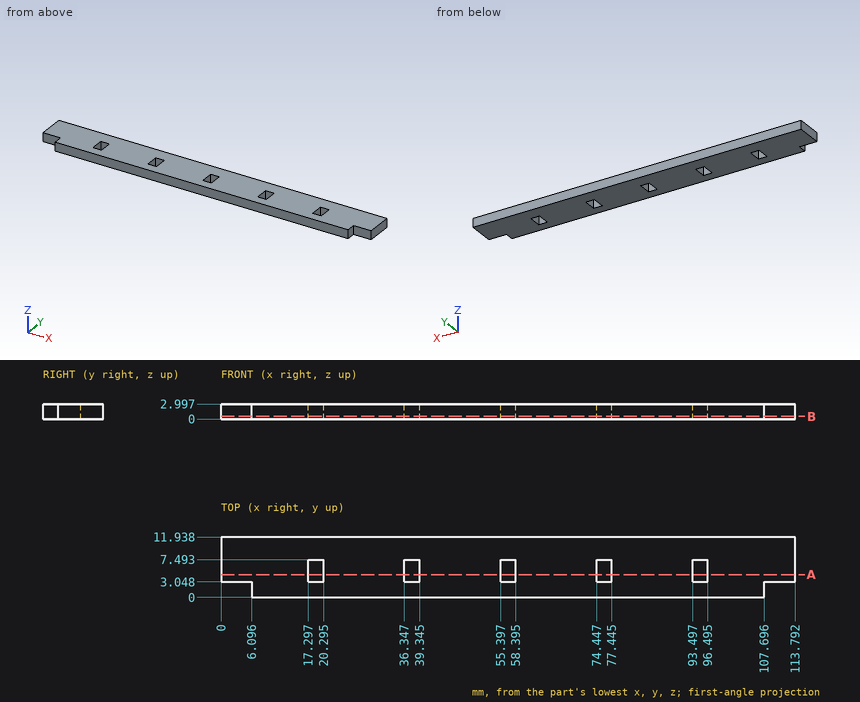
Here's the drawing with two shaded views (mm, measured from the low corner). I have some questions. Give positions to 0.01 mm unless a question says otherwise; leave off trailing zeros. Loops run counter-clockwise (first coordinate to the right, second up) from the corner with the lowest first, then second, coordinate; pieces in that order, holes last. Notation, with made-up numbers: M 43.5,23 L 64.5,23 A33 cw 64.5,62 Z; hole C 23,73 d7. An arc over 180 degrees is marked long. One line per item, written item: value.
1) Please list where these lines run through material, in increasing order: line 1 (X direction, y = 3.75, z = 1.15) (1 decimal); line 2 (Y direction, x = 19.5, z = 1.1); line 3 (X direction, y = 2, z = 2.05).
Geometry check:
line 1: x = 0 to 17.3, 20.3 to 36.3, 39.3 to 55.4, 58.4 to 74.4, 77.4 to 93.5, 96.5 to 113.8
line 2: y = 0 to 3.05, 7.49 to 11.94
line 3: x = 6.1 to 107.7
2) Imagine slicing it at B-B on z = 0.55. Write out the boundary of the cut face in (x, y) (1 decimal).
Geometry check:
outline: M 0,3 L 6.1,3 L 6.1,0 L 107.7,0 L 107.7,3 L 113.8,3 L 113.8,11.9 L 0,11.9 Z; hole M 17.3,3 L 20.3,3 L 20.3,7.5 L 17.3,7.5 Z; hole M 36.3,3 L 39.3,3 L 39.3,7.5 L 36.3,7.5 Z; hole M 55.4,3 L 58.4,3 L 58.4,7.5 L 55.4,7.5 Z; hole M 74.4,3 L 77.4,3 L 77.4,7.5 L 74.4,7.5 Z; hole M 93.5,3 L 96.5,3 L 96.5,7.5 L 93.5,7.5 Z
3) Imagine slicing it at A-A on y = 4.5. Write out the boundary of the cut face in (x, z) (1 decimal).
Geometry check:
outline: M 0,0 L 17.3,0 L 17.3,3 L 0,3 Z; M 20.3,0 L 36.3,0 L 36.3,3 L 20.3,3 Z; M 39.3,0 L 55.4,0 L 55.4,3 L 39.3,3 Z; M 58.4,0 L 74.4,0 L 74.4,3 L 58.4,3 Z; M 77.4,0 L 93.5,0 L 93.5,3 L 77.4,3 Z; M 96.5,0 L 113.8,0 L 113.8,3 L 96.5,3 Z
4) I'm going to push flat-ended pins straight in: pin 1 (1.5 mm diameter, centred on y = 8, z = 2.5, fed in from -X); pin 2 (1.5 mm diameter, centred on x = 4.5, z = 1, fed in from -Y). Where does each tip first touch, or does it pass through?
Geometry check:
pin 1: stops at x = 0
pin 2: stops at y = 3.05
